Source: CAD feature listing. Evaluate the final solid. Frame: model axes, mm. A direction names the side the tool comes from. Round coordinates to 2 decimals unless told otherwise and drop trailing zeros. Order: outer loops, then holes, each group sorted by start corner. A loop starts at its lowest first (then second) coordinate and runs counter-clockwise, first axis right, second up. Notation, with made-up numbers: (23.25, -29) -> (51.25, -29) arc R18 cw to (51.25, 3) -> close; hole circle Ø2 at (-2.5, 3). An arc over 180 degrees is marked (long way). Write item = value, one per line. Start each with the question number.
(1) Draft query along Y for faces 1 (the face through (-38.1, -15, 6)), 2 (the face through (7.827, -4.624, 6.439)), 3 (the face through (32, -25.4, 6)). Return one class per face: released by +Y, released by -Y, zero draft, split by the parting line, or undercut.
(2) Ray query, line 1 (X direction, y = -9.25, z = 11); line 2 (X direction, y = -4.5, z = 2.75); line 3 (X direction, y = -22.75, z = 7.5). Return the intervals inside material, ascending.
(3) Cut plane C-C on x = 24.5. Return the cut outline in (y, z), then the cut area to 3 significant figures.
(4) Reachability of faces 4 (the face through (-32, -25.4, 6)), 5 (the face through (25.4, -22, 6)) from +Z, -Z, +X, -X, +Y, -Y: full face, straight path, thin tool, end or side. Return the list, or none.
(5) Cut plane A-A on y = -16. Return the cut outline in (x, z).
(6) Cut plane B-B on y = -8.75. Return the cut outline in (x, z), then the cut area to 3 significant figures.
(7) Cut plane D-D on z = 5.5. Give the number of separate pieces and of enclosed holes in the cut face, then the cut area to 3 significant figures.
from build123d import *

# Parameters (mm, degrees)
SKETCH1_R           = 4.064
BOSS_EXTRUDE1_DEPTH = 12.7
SKETCH2_R           = 1.6999966
SKETCH2_R_2         = 1.7
CUT_EXTRUDE1_DEPTH  = 48.519048812


with BuildPart() as part:
    # Sketch1 → Boss-Extrude1 (new body)
    with BuildSketch(Plane.XY):
        Polygon((0, 0), (-38.1, 0), (-38.1, -25.4), (-25.4, -25.4), (-25.4, -19.05), (-12.7, -12.7), (0, -12.7), align=None)
        with Locations((-26.924, -9.525)):
            Circle(SKETCH1_R, mode=Mode.SUBTRACT)
    boss_extrude1 = extrude(amount=BOSS_EXTRUDE1_DEPTH)

    # Mirror1: Boss-Extrude1 across plane
    add(boss_extrude1.mirror(Plane(origin=(0, -12.7, 12.7), x_dir=(0, 0, 1), z_dir=(-1, 0, 0))))

    # Sketch2 → Cut-Extrude1 (cut, through all)
    with BuildSketch(Plane.XY.offset(12.7)):
        with Locations((-9.525, -4.699)):
            Circle(SKETCH2_R)
        with Locations((9.525, -4.699)):
            Circle(SKETCH2_R_2)
        with BuildLine():
            Line((-38.1, -4.011499418), (-38.1, 0))
            Line((-38.1, 0), (-34.28223801, 0))
            ThreePointArc((-34.28223801, 0), (-36.246656766, -1.952894173), (-38.1, -4.011499418))
        make_face()
        with BuildLine():
            Line((34.28223801, 0), (38.1, 0))
            Line((38.1, 0), (38.1, -4.011499418))
            ThreePointArc((38.1, -4.011499418), (36.246656766, -1.952894173), (34.28223801, 0))
        make_face()
    extrude(amount=-CUT_EXTRUDE1_DEPTH, mode=Mode.SUBTRACT)


solid = part.part
Evaluation:
q1.face_1 = zero draft
q1.face_2 = undercut
q1.face_3 = released by -Y
q2.line_1 = -38.1 to -30.98, -22.87 to 22.87, 30.98 to 38.1
q2.line_2 = -38.1 to -11.21, -7.84 to 7.84, 11.21 to 38.1
q2.line_3 = -38.1 to -25.4, 25.4 to 38.1
q3.outline = (-18.6, 0) -> (-12.79, 0) -> (-12.79, 12.7) -> (-18.6, 12.7) -> close; (-6.26, 0) -> (0, 0) -> (0, 12.7) -> (-6.26, 12.7) -> close
q3.area = 153 mm^2
q4.face_4 = +Z, -Z, +X, -X, -Y
q4.face_5 = +Z, -Z, -Y
q5.outline = (-38.1, 0) -> (-19.3, 0) -> (-19.3, 12.7) -> (-38.1, 12.7) -> close; (19.3, 0) -> (38.1, 0) -> (38.1, 12.7) -> (19.3, 12.7) -> close
q6.outline = (-38.1, 0) -> (-30.91, 0) -> (-30.91, 12.7) -> (-38.1, 12.7) -> close; (-22.93, 0) -> (22.93, 0) -> (22.93, 12.7) -> (-22.93, 12.7) -> close; (30.91, 0) -> (38.1, 0) -> (38.1, 12.7) -> (30.91, 12.7) -> close
q6.area = 765 mm^2
q7.separate_pieces = 1
q7.enclosed_holes = 4
q7.area = 1,230 mm^2
